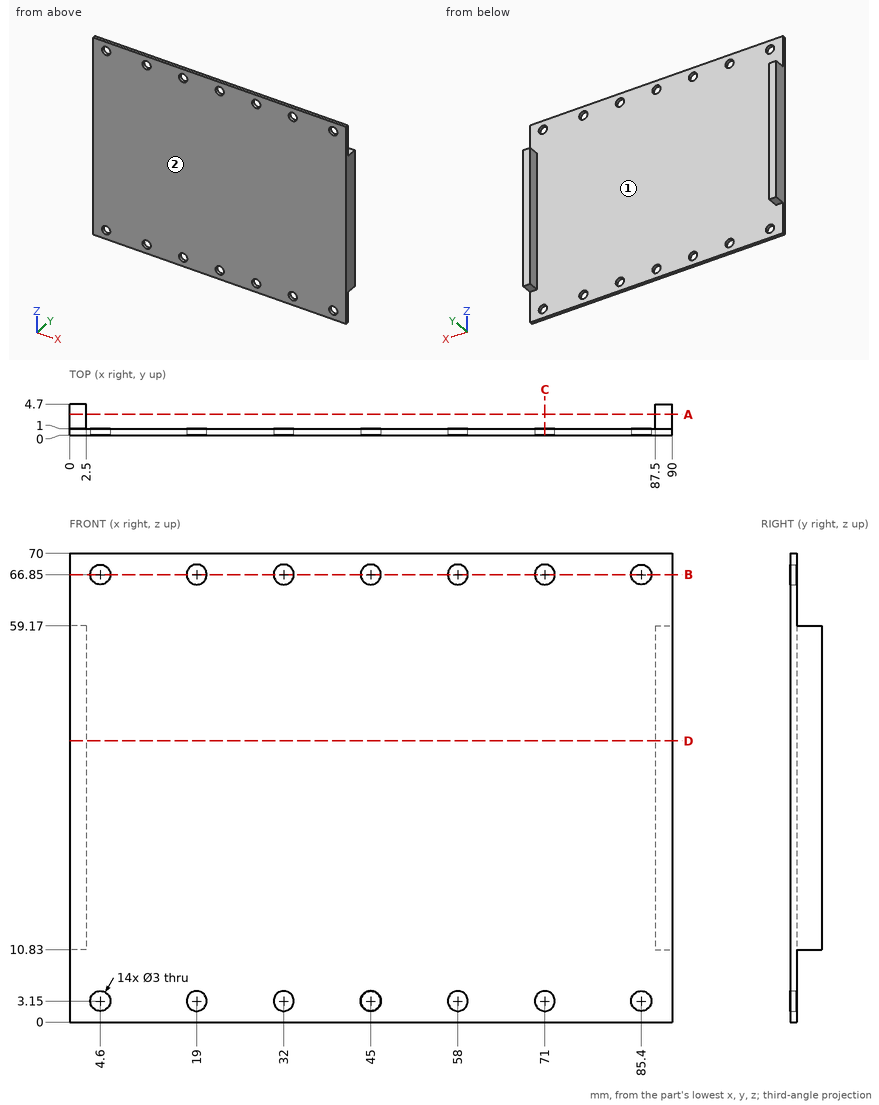
Study the drawing (mm; zero at the part's minimum x, y, z) and answer. Give positions to 0.01 mm unless a question says otherwise; leave off trailing zeros. Write each loop counter-clockwise with the first axis right and the second up, starting at its lowest first coordinate (ties: lowest second). Pieces come first, ordered by that corner, then holes. Notation, with made-up numbers: (36.5, 80) - (68.5, 80) arc R20 ccw to (68.5, 110) - close; hole circle Ø2 at (46.25, 51). An arc over 180 degrees is marked (long way). Use a Markdown table: item, result.
1. Section A-A on y = 3.15 is taken. Write down the section's boundary in (x, z).
Values follow:
| item | result |
|---|---|
| outline | (0, 10.83) - (2.5, 10.83) - (2.5, 59.17) - (0, 59.17) - close; (87.5, 10.83) - (90, 10.83) - (90, 59.17) - (87.5, 59.17) - close |
2. Each of these flat-tipped pins is pushed along its axis until it touches: P1, Ø0.8, axis at x = 1, y = 3, coming from the +Z side; P2, Ø5, axis at x = 4.6, z = 66.85, coming from the +Y side; P3, Ø3.5, axis at x = 85.4, z = 3.15, coming from the -Y side; P4, Ø2, axis at x = 89, y = 2.5, coming from the -Z side. Where does it stop, or does it pass through?
Values follow:
| item | result |
|---|---|
| P1 | stops at z = 59.17 |
| P2 | stops at y = 1 |
| P3 | stops at y = 0 |
| P4 | stops at z = 10.83 |
3. Find the intervals of material crossed by probe 1 along Z at (x, y) = (71, 0.4); probe 2 along X at (y, z) = (1.5, 19.5); probe 3 along Y at (x, z) = (77.5, 12), in increasing order. Write a range as from..to.
Values follow:
| item | result |
|---|---|
| probe 1 | z = 0..1.65, 4.65..65.35, 68.35..70 |
| probe 2 | x = 0..2.5, 87.5..90 |
| probe 3 | y = 0..1 |
4. Section B-B on z = 66.85 is taken. Count the separate pieces of the cut face and the enclosed holes in it, plus the area to 3 significant figures.
Values follow:
| item | result |
|---|---|
| separate pieces | 8 |
| enclosed holes | 0 |
| area | 69.0 mm² |
5. Section C-C on x = 71 is taken. Write down the section's boundary in (y, z).
Values follow:
| item | result |
|---|---|
| outline | (0, 0) - (1, 0) - (1, 1.65) - (0, 1.65) - close; (0, 4.65) - (1, 4.65) - (1, 65.35) - (0, 65.35) - close; (0, 68.35) - (1, 68.35) - (1, 70) - (0, 70) - close |
6. For a pull along X with two mould halves and no side action, classify the marked faces 1 and 2 as released by +X, released by -X, zero draft, split by the parting line, or undercut.
Values follow:
| item | result |
|---|---|
| face 1 | undercut |
| face 2 | zero draft |
7. Section D-D on z = 42 is taken. Write down the section's boundary in (x, y).
Values follow:
| item | result |
|---|---|
| outline | (0, 0) - (90, 0) - (90, 4.7) - (87.5, 4.7) - (87.5, 1) - (2.5, 1) - (2.5, 4.7) - (0, 4.7) - close |
